Design review of the part built by this model. Coordinates are the model's own, in mm. A direction names the side the tool comes from. Give positions to 0.01 mm unless a question says otherwise; leave off trailing zeros. Loops run counter-clockwise (first coordinate to the right, second up) from the corner with the lowest first, then second, coordinate; pieces in that order, holes last. Notation, with made-up numbers: (-39, 68) - (20, 68) arc R18 ccw to (20, 96) - close; hole circle Ø7 at (-16, 73.25). An arc over 180 degrees is marked (long way). Put each result on its own line as item: value. Start each with the question number.
```python
from build123d import *

# Parameters (mm, degrees)
F0_R     = 2.54
F0_R_2   = 15.875
F1_DEPTH = 6.35
F0_R_3   = 12.192
F2_DEPTH = 7.62
F3_DEPTH = 25.4


with BuildPart() as f1:
    # F0 (on Front) → F1 (new body)
    with BuildSketch(Plane.XZ):
        with BuildLine():
            ThreePointArc((28.575, 0), (20.205576, 20.205576), (0, 28.575))
            ThreePointArc((0, 28.575), (-20.205576, 20.205576), (-28.575, 0))
            ThreePointArc((-28.575, 0), (-20.205576, -20.205576), (0, -28.575))
            ThreePointArc((0, -28.575), (20.205576, -20.205576), (28.575, 0))
        make_face()
        with Locations((-11.90625, -20.62223)):
            Circle(F0_R, mode=Mode.SUBTRACT)
        with Locations((11.90625, -20.62223)):
            Circle(F0_R, mode=Mode.SUBTRACT)
        with Locations((-23.8125, 0)):
            Circle(F0_R, mode=Mode.SUBTRACT)
        with Locations((-11.90625, 20.62223)):
            Circle(F0_R, mode=Mode.SUBTRACT)
        Circle(F0_R_2, mode=Mode.SUBTRACT)
        with Locations((23.8125, 0)):
            Circle(F0_R, mode=Mode.SUBTRACT)
        with Locations((11.90625, 20.62223)):
            Circle(F0_R, mode=Mode.SUBTRACT)
    extrude(amount=F1_DEPTH)

    # F0 (on Front) → F2 (join)
    with BuildSketch(Plane.XZ):
        Circle(F0_R_2)
        Circle(F0_R_3, mode=Mode.SUBTRACT)
    extrude(amount=F2_DEPTH)

    # F0 (on Front) → F3 (join)
    with BuildSketch(Plane.XZ):
        Circle(F0_R_3)
        Polygon((0, 7.086949), (6.536717, 3.637514), (6.536717, -3.637514), (0, -7.086949), (-6.315683, -3.440588), (-6.315683, 3.440588), align=None, mode=Mode.SUBTRACT)
    extrude(amount=F3_DEPTH)


solid = f1.part
```
Item 1: Consider section C-C (x = 11.5). State the section outline as (y, z) points, plus the area to 3 significant figures.
Item 2: Consider section B-B (x = 4.5). State the section outline as (y, z) points.
Item 3: Consider section A-A (y = -11.25). State the section outline as (x, z) points, plus the area to 3 significant figures.
Item 4: Consider section D-D (y = -4.25). Count the separate pieces of the cut face and the enclosed holes in it, plus the area to 3 significant figures.
Item 5: For P1, Ø8, axis at y = -12, z = 1.5, coming from the -X side; P2, Ø2, axis at x = 0, z = -14, coming from the -Y side; P3, Ø2, axis at x = -1, z = 17.5, coming from the -Y side, all flat-tipped, find the tip position at first contact; note any pin that passes through.
Item 6: Mouldability with a two-part tool opening along X and no side actions: class faces 4 (the flat face through (-7, 0, 0)), 5 (the cylindrical face through (-1.587, -16.386, 12.088)), 6 (the cylindrical face through (-21.466, -3.131, -0.973)) as pulls with the +X half, pulls with the -X half, needs draft (parallel to the pull), parting line crosses it, or undercut.
Item 7: For L1, parallel to X at y = -2, z = 21; L2, parallel to Y at x = -9.5, z = -22.5; L3, parallel to Z at x = -24.5, y = -4, list the stretches that pass through material, from the lowest coordinate up. Write a range as from..to.
Item 8: Machinability: for faces 1 (the cylindrical face through (-3.441, -6.976, -15.497)), 2 (the flat face through (-6.316, -13, 0)), 3 (the flat face through (-3, -25.4, 6)), which of the approach directions +Z, -Z, +X, -X, +Y, -Y give a long, thin tool a straight path to every point of the face, cutting with its end or side? Answer none if there is none.
Geometry says:
1. outline: (-25.4, -4.05) - (-7.62, -4.05) - (-7.62, -10.94) - (-6.35, -10.94) - (-6.35, -18.11) - (0, -18.11) - (0, 18.11) - (-6.35, 18.11) - (-6.35, 10.94) - (-7.62, 10.94) - (-7.62, 4.05) - (-25.4, 4.05) - close; (-6.35, -26.16) - (0, -26.16) - (0, -23.13) - (-6.35, -23.13) - close; (-6.35, 23.13) - (0, 23.13) - (0, 26.16) - (-6.35, 26.16) - close
1. area: 440 mm2
2. outline: (-25.4, -11.33) - (-7.62, -11.33) - (-7.62, -15.22) - (-6.35, -15.22) - (-6.35, -28.22) - (0, -28.22) - (0, -4.71) - (-25.4, -4.71) - close; (-25.4, 4.71) - (0, 4.71) - (0, 28.22) - (-6.35, 28.22) - (-6.35, 15.22) - (-7.62, 15.22) - (-7.62, 11.33) - (-25.4, 11.33) - close
3. outline: circle Ø24.38 at (0, 0); hole (-6.32, -3.44) - (0, -7.09) - (6.54, -3.64) - (6.54, 3.64) - (0, 7.09) - (-6.32, 3.44) - close
3. area: 330 mm2
4. separate pieces: 1
4. enclosed holes: 7
4. area: 2,310 mm2
5. P1: stops at x = -12.19
5. P2: stops at y = -7.62
5. P3: stops at y = -6.35
6. face 4: needs draft
6. face 5: parting line crosses it
6. face 6: undercut
7. L1: x = -19.38..-14.42, -9.39..9.39, 14.42..19.38
7. L2: y = -6.35..0
7. L3: z = -14.71..-2.45, 2.45..14.71
8. face 1: -Y
8. face 2: +Y, -Y
8. face 3: +Z, -Z, +X, -X, -Y
